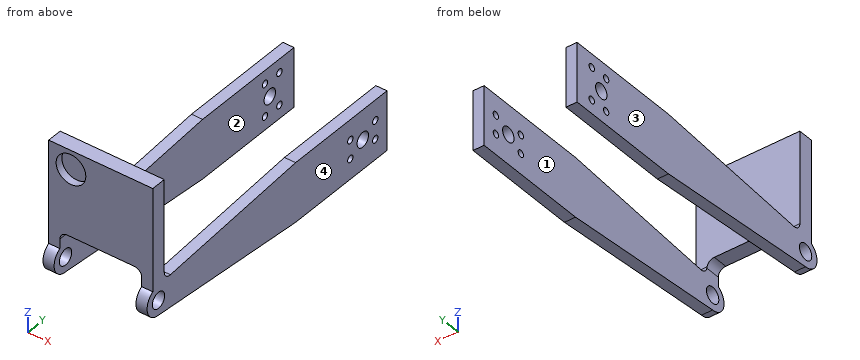
Autodesk Inventor part; units mm, degrees
ref_plane "YZ Plane" through (0, 0, 0) normal (1, 0, 0) x (0, 1, 0)
ref_plane "XZ Plane" through (0, 0, 0) normal (0, 1, 0) x (-1, 0, 0)
ref_plane "XY Plane" through (0, 0, 0) normal (0, 0, 1) x (1, 0, 0)
sketch "Sketch1" plane through (0, 0, 0) normal (1, 0, 0) x (0, 1, 0)
  line L0 (0, 0) -> (127, 0)
  line L1 (127, 0) -> (127, -25.4)
  line L2 (127, -25.4) -> (0, -25.4)
  line L3 (0, -25.4) -> (0, 0)
  line L4 (0, -6.35) -> (0, -19.05)
  line L5 (0, -6.35) -> (76.2, 0)
  line L6 (0, -19.05) -> (76.2, -25.4)
  dimension "d0" = 127
  dimension "d1" = 25.4
  dimension "d18" = 12.7
  dimension "d19" = 6.35
  dimension "d20" = 50.8
  dimension "d21" = 50.8
ref_plane "Work Plane1" through (44.5262, 0, 0) normal (1, 0, 0) x (0, 0, -1)
sketch "Sketch2" plane through (44.5262, 0, 0) normal (1, 0, 0) x (0, 0, -1)
  line L0 (0, 127) -> (0, 0)
  line L1 (0, 0) -> (25.4, 0)
  line L2 (25.4, 0) -> (25.4, 127)
  line L3 (25.4, 127) -> (0, 127)
  line L4 (0, 0) -> (25.4, 0)
  circle A0 centre (12.7, 0) radius 6.35
  dimension "d5" = 25.4
  dimension "d6" = 12.7
  dimension "d7" = 12.7
  dimension "d8" = 0
extrude "Extrusion2" add sketch "Sketch2" against normal blind 44.5262 contours A0 L1 | L1 A0
ref_plane "Work Plane2" through (44.5262, 0, 0) normal (1, 0, 0) x (0, 0, -1)
extrude "Extrusion3" add sketch "Sketch1" along normal blind 44.5262 contours L0 L1 L2 L6 L3 L5
sketch "Sketch4" plane through (0, 0, 0) normal (-1, 0, 0) x (0, 0, 1)
  arc A0 (-19.05, 0) -> (-6.35, 0) centre (-12.7, 0) ccw
  line L0 (0, 76.2) -> (-6.35, 0)
  line L1 (0, 127) -> (0, 76.2)
  line L2 (-25.4, 127) -> (0, 127)
  line L3 (-25.4, 76.2) -> (-25.4, 127)
  line L4 (-19.05, 0) -> (-25.4, 76.2)
  point P0 (0, 0)
hole "Hole2" at (0, 0, -12.7) direction (1, 0, 0) diameter 6.858 end through all
sketch "Sketch5" plane through (0, 0, 0) normal (-1, 0, 0) x (0, 0, 1)
  circle A0 centre (-12.7, 0) radius 3.429
  line L0 (0, 76.2) -> (-6.35, 0)
  line L1 (0, 127) -> (0, 76.2)
  line L2 (-25.4, 127) -> (0, 127)
  line L3 (-25.4, 76.2) -> (-25.4, 127)
  line L4 (-19.05, 0) -> (-25.4, 76.2)
  line L5 (-7.6835, 3.175) -> (36.7665, 3.175)
  line L6 (36.7665, 3.175) -> (36.7665, -3.175)
  line L7 (36.7665, -3.175) -> (-7.6835, -3.175)
  line L8 (-7.6835, -3.175) -> (-7.6835, 3.175)
  arc A1 (-19.05, 0) -> (-6.35, 0) centre (-12.7, 0) ccw
  point P0 (0, 0)
  dimension "d31" = 44.45
  dimension "d32" = 6.35
  dimension "d35" = 127
  dimension "d36" = 123.825
  dimension "d95" = 6.858
  dimension "d96" = 5.0165
extrude "Extrusion4" add sketch "Sketch5" against normal blind 44.5262 contours L5 L6 L7 A1 L0 | L0 A1 L7 L8 L5
sketch "Sketch8" plane through (0, 76.2, -25.4) normal (0, 0, -1) x (-1, 0, 0)
  line L0 (0, 0) -> (0, 50.8)
  line L1 (0, 50.8) -> (-44.5262, 50.8)
  line L2 (-44.5262, 0) -> (-44.5262, 50.8)
  line L3 (0, 0) -> (-44.5262, 0)
  line L4 (0, -76.2) -> (0, 0)
  line L5 (0, 0) -> (-44.5262, 0)
  line L6 (-44.5262, -76.2) -> (-44.5262, 0)
  line L7 (0, 50.8) -> (-44.5262, 50.8)
  line L8 (-39.7637, 50.8) -> (-4.7625, 50.8)
  line L9 (-4.7625, 50.8) -> (-4.7625, -98.425)
  line L10 (-4.7625, -98.425) -> (-39.7637, -98.425)
  line L11 (-39.7637, -98.425) -> (-39.7637, 50.8)
  line L12 (0, -76.2) -> (-44.5262, -76.2)
  point P0 (0, -76.2)
  dimension "d41" = 44.5262
  dimension "d43" = 35.0012
  dimension "d44" = 4.7625
  dimension "d45" = 149.225
extrude "Extrusion5" cut sketch "Sketch8" against normal blind 25.4 contours L9 L12 L11 L3 | L3 L11 L1 L9 | L9 L10 L11 L12
fillet "Fillet1" radius 3.175 2 edges at (39.7637, 0, 0) (4.7625, 0, 0)
fillet "Fillet2" radius 3.175 2 edges at (2.3812, 3.175, -6.0854) (42.1449, 3.175, -6.0854)
sketch "Sketch9" plane through (0, 0, 0) normal (-1, 0, 0) x (0, 0, 1)
  line L0 (0, 76.2) -> (-5.7989, 6.6137)
  line L1 (0, 127) -> (0, 76.2)
  line L2 (-25.4, 127) -> (0, 127)
  line L3 (-25.4, 76.2) -> (-25.4, 127)
  line L4 (-19.05, 0) -> (-25.4, 76.2)
  circle A0 centre (-12.7, 0) radius 3.429
  circle A1 centre (-12.7, 114.8637) radius 8
  line L5 (-19.6282, 118.8637) -> (-5.7718, 118.8637)
  line L6 (-5.7718, 118.8637) -> (-5.7718, 110.8637)
  line L7 (-5.7718, 110.8637) -> (-19.6282, 110.8637)
  line L8 (-19.6282, 110.8637) -> (-19.6282, 118.8637)
  arc A2 (-19.05, 0) -> (-7.2007, -3.175) centre (-12.7, 0) ccw
  line L9 (36.7665, -3.175) -> (-7.2007, -3.175)
  line L10 (36.7665, 3.175) -> (36.7665, -3.175)
  line L11 (-2.6348, 3.175) -> (36.7665, 3.175)
  arc A3 (-5.7989, 6.6137) -> (-2.6348, 3.175) centre (-2.6348, 6.35) ccw
  point P0 (0, 0)
  dimension "d50" = 16
  dimension "d51" = 25.4
  dimension "d52" = 12.7
  dimension "d53" = 8
  dimension "d54" = 4
hole "Hole3" at (0, 118.8637, -19.6282) at (0, 110.8637, -19.6282) at (0, 118.8637, -5.7718) at (0, 110.8637, -5.7718) direction (1, 0, 0) diameter 2.9718 depth 25.4 tip angle 118
sketch "Sketch10" plane through (44.5262, 0, 0) normal (1, 0, 0) x (0, 0, -1)
  line L0 (19.05, 0) -> (25.4, 76.2)
  line L1 (25.4, 76.2) -> (25.4, 127)
  line L2 (25.4, 127) -> (0, 127)
  line L3 (0, 127) -> (0, 76.2)
  line L4 (0, 76.2) -> (5.7989, 6.6137)
  circle A0 centre (12.7, 0) radius 3.429
  circle A1 centre (12.7, 113.546) radius 8
  line L5 (16.7, 106.6178) -> (8.7, 106.6178)
  line L6 (8.7, 106.6178) -> (8.7, 120.4742)
  line L7 (8.7, 120.4742) -> (16.7, 120.4742)
  line L8 (16.7, 120.4742) -> (16.7, 106.6178)
  arc A2 (7.2007, -3.175) -> (19.05, 0) centre (12.7, 0) ccw
  arc A3 (2.6348, 3.175) -> (5.7989, 6.6137) centre (2.6348, 6.35) ccw
  line L9 (2.6348, 3.175) -> (-36.7665, 3.175)
  line L10 (-36.7665, 3.175) -> (-36.7665, -3.175)
  line L11 (-36.7665, -3.175) -> (7.2007, -3.175)
  point P0 (0, 0)
  dimension "d62" = 16
  dimension "d63" = 25.4
  dimension "d64" = 12.7
  dimension "d65" = 8
  dimension "d66" = 4
hole "Hole4" at (44.5262, 106.6178, -16.7) at (44.5262, 106.6178, -8.7) at (44.5262, 120.4742, -8.7) at (44.5262, 120.4742, -16.7) direction (-1, 0, 0) diameter 2.9718 depth 25.4 tip angle 118
sketch "Sketch11" plane through (0, -3.175, -7.2007) normal (0, -1, 0) x (1, 0, 0)
  line L0 (4.7625, 0) -> (4.7625, 4.0257)
  arc A0 (7.9375, 7.2007) -> (4.7625, 4.0257) centre (7.9375, 4.0257) ccw
  line L1 (7.9375, 7.2007) -> (36.5887, 7.2007)
  arc A1 (39.7637, 4.0257) -> (36.5887, 7.2007) centre (36.5887, 4.0257) ccw
  line L2 (39.7637, 4.0257) -> (39.7637, 0)
  line L3 (44.5262, 43.9672) -> (44.5262, 0)
  line L4 (0, 43.9672) -> (44.5262, 43.9672)
  line L5 (0, 43.9672) -> (0, 0)
  line L6 (44.5262, 0) -> (39.7637, 0)
  line L7 (4.7625, 0) -> (0, 0)
  point P0 (0, 7.2007)
  point P1 (9.525, 35.8392)
  dimension "d74" = 8.128
  dimension "d75" = 44.5262
  dimension "d97" = 9.525
hole "Hole5" at (9.525, -3.175, 28.6385) direction (0, 1, 0) diameter 12.7 depth 3.175
sketch "Sketch12" plane through (44.5262, 0, 0) normal (1, 0, 0) x (0, 0, -1)
  circle A0 centre (8.7, 120.4742) radius 1.4859
  circle A1 centre (16.7, 106.6178) radius 1.4859
  circle A2 centre (8.7, 106.6178) radius 1.4859
  circle A3 centre (16.7, 120.4742) radius 1.4859
  line L0 (19.05, 0) -> (25.4, 76.2)
  line L1 (25.4, 76.2) -> (25.4, 127)
  line L2 (25.4, 127) -> (0, 127)
  line L3 (0, 127) -> (0, 76.2)
  line L4 (0, 76.2) -> (5.7989, 6.6137)
  circle A4 centre (12.7, 0) radius 3.429
  arc A5 (7.2007, -3.175) -> (19.05, 0) centre (12.7, 0) ccw
  arc A6 (2.6348, 3.175) -> (5.7989, 6.6137) centre (2.6348, 6.35) ccw
  line L5 (2.6348, 3.175) -> (-36.7665, 3.175)
  line L6 (-36.7665, 3.175) -> (-36.7665, -3.175)
  line L7 (-36.7665, -3.175) -> (7.2007, -3.175)
  point P0 (0, 0)
  point P1 (12.7, 113.546)
  dimension "d84" = 25.4
  dimension "d85" = 12.7
  dimension "d86" = 13.8564
  dimension "d87" = 6.9282
hole "Hole6" at (44.5262, 113.546, -12.7) direction (-1, 0, 0) diameter 6.35 end through all
equation "\"d19\" = -0.5 * d18 + 0.5 * d1"
equation "\"d21\" = d20"
equation "\"d7\" = 0.5 * d5"
equation "\"d36\" = d35 - 0.5 * d32"
equation "\"d44\" = -0.5 * d43 + 0.5 * d41"
equation "\"d52\" = 0.5 * d51"
equation "\"d54\" = 0.5 * d53"
equation "\"d64\" = 0.5 * d63"
equation "\"d66\" = 0.5 * d65"
properties part number "WheelIntakeMount3.0"
Source: CAD feature listing. Evaluate the final solid. Frame: model axes, mm. Face numbers are marked on the shaded views. Coordinates: 2 decimals unless noted, no trailing zeros. Loops run counter-clockwise (first coordinate to the right, second up) from the corner with the lowest first, then second, coordinate; pieces in that order, holes last. Notation, with made-up numbers: (20, 45) -> (36, 45) arc R12 ccw to (36, 65) -> close; hole circle Ø5 at (46, -16). An arc over 180 degrees is marked (long way). Answer in a Markdown table with one row per item. Add a question column.
Q1. Contact query for flat-ended pins moving along their axis: pin 1 Ø2.5 at (x, y) = (41.5, 110.5) entering from +Z; pin 2 Ø7 at (x, y) = (24.5, 0) entering from -Z; pin 3 Ø14 at (x, z) = (12.5, 27) entering from -Y (3 decimals); pin 4 Ø9 at (y, z) = (0, -12.7) entering from -X. Output: stop coordinate, or through.
Q2. Section D-D on x = 29.5. Return the cut outline in (y, z) (1 decimal), and give its area (3 significant figures).
Q3. Ray query, line 1 along Y through (x, z) = (2.5, -12.5); line 2 along X through (y, z) = (21, -8); line 3 along Y through (x, z) = (29, 14.5) (3 decimals). Return the intervals inside material, ascending.
Q4. Section C-C on z = 21. Return the cut outline in (x, y) (3 decimals).
Q5. Section A-A on z = -12.7. Return the cut outline in (x, y), and give its area (3 significant figures).
Q6. Section B-B on y = 32. Return the cut outline in (x, z).
Q7. Pull-direction query (X, two-part tool) for the marked faces 1, 2, 3 and 4; classes: pulls with the +X half, pulls with the -X half, needs draft (parallel to the pull), parting line crosses it, or undercut.
Computed values:
| question | item | result |
|---|---|---|
| 1 | pin 1 | stops at z = 0 |
| 1 | pin 2 | stops at z = 0 |
| 1 | pin 3 | stops at y = -3.175 |
| 1 | pin 4 | stops at x = 0 |
| 2 | outline | (-3.2, 0) -> (3.2, 0) -> (3.2, 36.8) -> (-3.2, 36.8) -> close |
| 2 | area | 233 mm^2 |
| 3 | line 1 | y = -6.35 to -3.42, 3.42 to 110.38, 116.71 to 127 |
| 3 | line 2 | x = 0 to 4.76, 39.76 to 44.53 |
| 3 | line 3 | y = -3.175 to 3.175 |
| 4 | outline | (0, -3.175) -> (44.526, -3.175) -> (44.526, 3.175) -> (0, 3.175) -> close |
| 5 | outline | (0, -6.35) -> (4.76, -6.35) -> (4.76, -3.43) -> (0, -3.43) -> close; (0, 3.43) -> (4.76, 3.43) -> (4.76, 110.37) -> (0, 110.37) -> close; (0, 116.72) -> (4.76, 116.72) -> (4.76, 127) -> (0, 127) -> close; (39.76, -6.35) -> (44.53, -6.35) -> (44.53, -3.43) -> (39.76, -3.43) -> close; (39.76, 3.43) -> (44.53, 3.43) -> (44.53, 110.37) -> (39.76, 110.37) -> close; (39.76, 116.72) -> (44.53, 116.72) -> (44.53, 127) -> (39.76, 127) -> close |
| 5 | area | 1,140 mm^2 |
| 6 | outline | (0, -21.72) -> (4.76, -21.72) -> (4.76, -3.68) -> (0, -3.68) -> close; (39.76, -21.72) -> (44.53, -21.72) -> (44.53, -3.68) -> (39.76, -3.68) -> close |
| 7 | face 1 | undercut |
| 7 | face 2 | undercut |
| 7 | face 3 | pulls with the -X half |
| 7 | face 4 | pulls with the +X half |
